```python
from build123d import *

# Parameters (mm, degrees)
F0_W     = 32
F0_H     = 32
F1_DEPTH = 20
F4_W     = 32
F4_H     = 32
F4_R     = 4
F5_DEPTH = 4


# Not quite as in the source:
# - the program builds the solid bodies; features that only make, move or delete a surface that nothing else refers to are left out


with BuildPart() as f1:
    # F0 (on Top) → F1 (new body)
    with BuildSketch(Plane.XY):
        with Locations((21.8166250885, -5.5067900717)):
            Rectangle(F0_W, F0_H)
    extrude(amount=F1_DEPTH)

    # F4 (on face) → F5 (join)
    with BuildSketch(Plane.XY.offset(20)):
        with Locations((21.8166250885, -5.5067900717)):
            Rectangle(F4_W, F4_H)
        with Locations((13.8166250885, -13.5067900717)):
            Circle(F4_R, mode=Mode.SUBTRACT)
        with Locations((29.8166250885, -13.5067900717)):
            Circle(F4_R, mode=Mode.SUBTRACT)
        with Locations((29.8166250885, 2.4932099283)):
            Circle(F4_R, mode=Mode.SUBTRACT)
    extrude(amount=F5_DEPTH)


solid = f1.part
```
Geometry: final body of the model. Coordinates: model frame, mm. A direction names the side the tool comes from. Coordinates: 2 decimals unless noted, no trailing zeros. Order: outer loops, then holes, each group sorted by start corner. A loop starts at its lowest first (then second) coordinate and runs counter-clockwise, first axis right, second up.
Item 1: Section query C-C (y = -14). Output: boundary loops of the cut face in (x, z).
Answer:
outline: (5.82, 0) - (37.82, 0) - (37.82, 24) - (33.79, 24) - (33.79, 20) - (25.85, 20) - (25.85, 24) - (17.79, 24) - (17.79, 20) - (9.85, 20) - (9.85, 24) - (5.82, 24) - close
Item 2: Section query B-B (x = 14). Output: boundary loops of the cut face in (y, z).
Answer:
outline: (-21.51, 0) - (10.49, 0) - (10.49, 24) - (-9.51, 24) - (-9.51, 20) - (-17.5, 20) - (-17.5, 24) - (-21.51, 24) - close
Item 3: Draft query along Y for faces 1 (the face through (22, 10.493, 12)), 2 (the face through (5.817, -6, 12)), 3 (the face through (31.967, -10.134, 21.972)). Return one class per face: released by +Y, released by -Y, zero draft, split by the parting line, or undercut.
Answer:
face 1: released by +Y
face 2: zero draft
face 3: undercut
Item 4: Material intervals for line 1 along Y through (x, z) = (30, 23.25); line 2 along X through (y, z) = (2.5, 21); line 3 along Z through (x, y) = (14, -15.5), sorted ascending.
Answer:
line 1: y = -21.51 to -17.5, -9.51 to -1.5, 6.49 to 10.49
line 2: x = 5.82 to 25.82, 33.82 to 37.82
line 3: z = 0 to 20
Item 5: Section query A-A (z = 22.75). Output: boundary loops of the cut face in (x, y), then the cut area to 3 significant figures.
Answer:
outline: (5.82, -21.51) - (37.82, -21.51) - (37.82, 10.49) - (5.82, 10.49) - close; hole circle Ø8 at (13.82, -13.51); hole circle Ø8 at (29.82, -13.51); hole circle Ø8 at (29.82, 2.49)
area: 873 mm2
Item 6: Contact query for a flat-ended pin moving along its axis: P1, Ø4, axis at x = 30.5, y = -13.5, coming from the +Z side. Output: stop coordinate, or through.
Answer:
P1: stops at z = 20
Item 7: Access query for faces 4 (the face through (30, -13, 20)), 5 (the face through (22, -5, 0)). Directions: +Z, -Z, +X, -X, +Y, -Y. A direction counts if a zero-diameter tool reaches every point of the face in a straight line with its end or side. Return the directions, or none.
Answer:
face 4: +Z
face 5: -Z, +X, -X, +Y, -Y
Item 8: Section query D-D (x = 32). Output: boundary loops of the cut face in (y, z).
Answer:
outline: (-21.51, 0) - (10.49, 0) - (10.49, 24) - (5.84, 24) - (5.84, 20) - (-0.86, 20) - (-0.86, 24) - (-10.16, 24) - (-10.16, 20) - (-16.86, 20) - (-16.86, 24) - (-21.51, 24) - close
